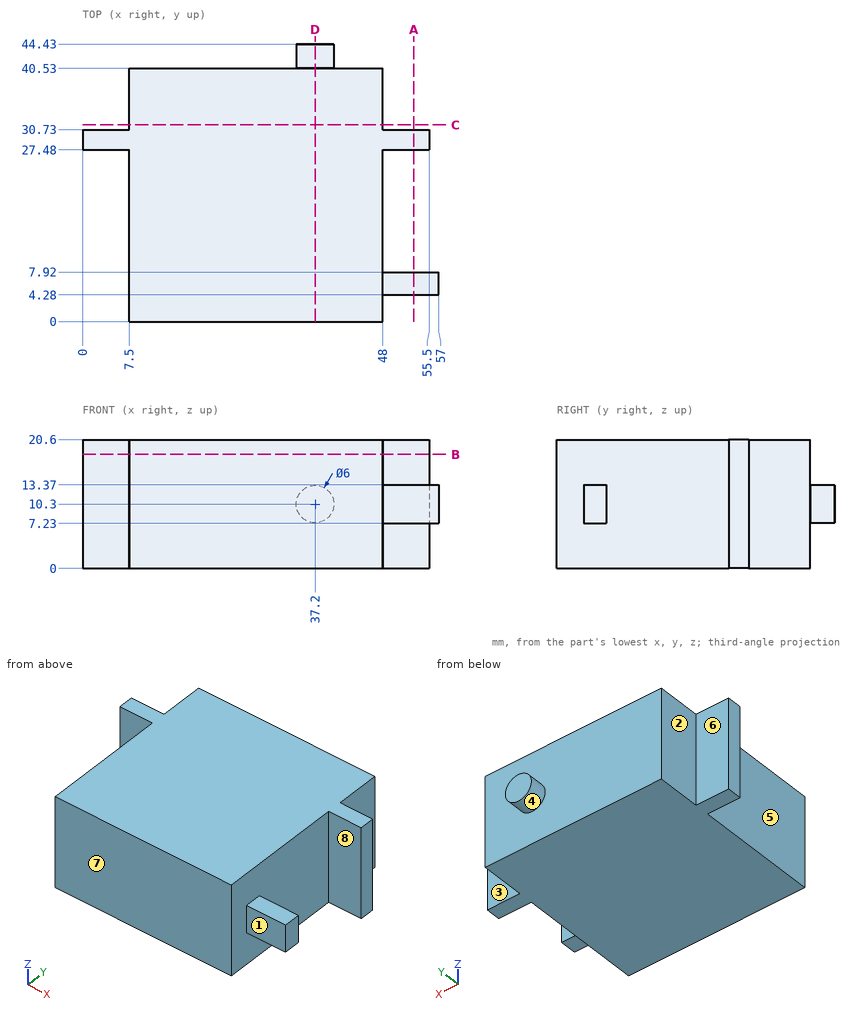
Can you work these out from the drawing? Everything is in mm from the part's minimum corner. A direction names the side the tool comes from. Coordinates: 2 decimals unless noted, no trailing zeros. Loops run counter-clockwise (first coordinate to the right, second up) from the corner with the lowest first, then second, coordinate; pieces in that order, holes last. Notation, with made-up numbers: (-39.5, 7) -> (-32.5, 7) arc R17 ccw to (-32.5, 26) -> close; hole circle Ø5 at (31.5, 12). An arc over 180 degrees is marked (long way). Return JSON: item names as keys, results as strings.
1) Thinking about a two-plate mould opening in Y: for the marked faces 6, 7 and 8, which applies, +Y half, -Y half, draft (parallel to the pull), parting line (faces both ways), or undercut?
Results below:
{"face 6": "+Y half", "face 7": "-Y half", "face 8": "undercut"}
2) For the marked faces 1, 2, 3, 4 and 5, which set-ups out of +Z, -Z, +X, -X, +Y, -Y let a thin tool reach every point of the face, with its end or its side?
Results below:
{"face 1": "+Z, -Z, +X, -Y", "face 2": "+Z, -Z, -X, +Y", "face 3": "+Z, -Z, +X, +Y", "face 4": "+Y", "face 5": "+Z, -Z, -X, -Y"}
3) If we section it at B-B, the plane z = 18.25: Write out the boundary of the cut face in (x, y).
Results below:
{"outline": "(0, 27.48) -> (7.5, 27.48) -> (7.5, 0) -> (48, 0) -> (48, 27.48) -> (55.5, 27.48) -> (55.5, 30.73) -> (48, 30.73) -> (48, 40.53) -> (7.5, 40.53) -> (7.5, 30.73) -> (0, 30.73) -> close"}
4) Will these pins go through, and if not, where does the flat tip stop? pin 1 (3.5 mm diameter, centred on y = 30, z = 9, fed in from +X); pin 2 (5 mm diameter, centred on y = 36, z = 9.5, fed in from +X); pin 3 (6 mm diameter, centred on y = 21.5, z = 6.5, fed in from -X); pin 4 (8 mm diameter, centred on x = 51, z = 15, fed in from -Y).
Results below:
{"pin 1": "x = 55.5", "pin 2": "x = 48", "pin 3": "x = 7.5", "pin 4": "y = 0"}
5) If we section it at D-D, the plane x = 37.2: Write out the boundary of the cut face in (y, z), then the cut area to 3 significant figures.
Results below:
{"outline": "(0, 0) -> (40.53, 0) -> (40.53, 7.3) -> (44.43, 7.3) -> (44.43, 13.3) -> (40.53, 13.3) -> (40.53, 20.6) -> (0, 20.6) -> close", "area": "858 mm²"}
6) If we section it at A-A, the plane x = 53: Write out the boundary of the cut face in (y, z).
Results below:
{"outline": "(4.28, 7.23) -> (7.92, 7.23) -> (7.92, 13.37) -> (4.28, 13.37) -> close; (27.48, 0) -> (30.73, 0) -> (30.73, 20.6) -> (27.48, 20.6) -> close"}
7) If we section it at C-C, the plane y = 31.5: Write out the boundary of the cut face in (x, z), then the cut area to 3 significant figures.
Results below:
{"outline": "(7.5, 0) -> (48, 0) -> (48, 20.6) -> (7.5, 20.6) -> close", "area": "834 mm²"}
8) I need wall thicknesses on line 1 (Y direction, x = 4, z = 5); line 2 (X direction, y = 4, z = 12.5); line 3 (Y direction, x = 21.5, z = 12.25). Which ranges of each line are inside material? Lowest first, please. Write a range as from..to.
Results below:
{"line 1": "27.48..30.73", "line 2": "7.5..48", "line 3": "0..40.53"}
